```python
from build123d import *

# Parameters (mm, degrees)
SKETCH1_W           = 120
SKETCH1_H           = 20
SKETCH1_W_2         = 25.5
SKETCH1_H_2         = 12.4
BOSS_EXTRUDE1_DEPTH = 6
SKETCH3_R           = 0.55
BOSS_EXTRUDE2_DEPTH = 3
SKETCH4_W           = 36
SKETCH4_H           = 20
BOSS_EXTRUDE3_DEPTH = 1.8
SKETCH5_R           = 3.4
CUT_EXTRUDE1_DEPTH  = 1.8
FILLET1_R           = 0.6


with BuildPart() as part:
    # Sketch1 → Boss-Extrude1 (new body)
    with BuildSketch(Plane(origin=(0, 0, 0), x_dir=(1, 0, 0), z_dir=(0, 1, 0))):
        with Locations((60, 10)):
            Rectangle(SKETCH1_W, SKETCH1_H)
        with BuildLine():
            Line((93.674922601, 11.942124585), (109.694736842, 13.386268507))
            ThreePointArc((109.694736842, 13.386268507), (113.4, 10), (109.694736842, 6.613731493))
            Line((109.694736842, 6.613731493), (93.674922601, 8.057875415))
            ThreePointArc((93.674922601, 8.057875415), (91.9, 10), (93.674922601, 11.942124585))
        make_face(mode=Mode.SUBTRACT)
        with Locations((17.75, 10)):
            Rectangle(SKETCH1_W_2, SKETCH1_H_2, mode=Mode.SUBTRACT)
    extrude(amount=BOSS_EXTRUDE1_DEPTH)

    # Sketch3 → Boss-Extrude2 (add)
    with BuildSketch(Plane.XZ):
        with Locations(Location((4.25, -10, 0), (0, 0, 270))):
            Circle(SKETCH3_R)
        with Locations(Location((31.25, -10, 0), (0, 0, 270))):
            Circle(SKETCH3_R)
    extrude(amount=BOSS_EXTRUDE2_DEPTH)

    # Sketch4 → Boss-Extrude3 (add)
    with BuildSketch(Plane(origin=(0, 6, 0), x_dir=(1, 0, 0), z_dir=(0, 1, 0))):
        with Locations((102, 10)):
            Rectangle(SKETCH4_W, SKETCH4_H)
    extrude(amount=-BOSS_EXTRUDE3_DEPTH)

    # Sketch5 → Cut-Extrude1 (cut)
    with BuildSketch(Plane.XZ.offset(-4.2)):
        with Locations(Location((110, -10, 0), (0, 0, 270))):
            Circle(SKETCH5_R)
    extrude(amount=-CUT_EXTRUDE1_DEPTH, mode=Mode.SUBTRACT)

    # Fillet1
    fillet1_edges = [part.edges().sort_by_distance(p)[0] for p in [
        (120, 6, -10),
        (60, 6, -20),
        (0, 6, -10),
        (60, 0, -20),
        (120, 0, -10),
        (60, 0, 0),
        (0, 0, -10),
        (60, 6, 0),
    ]]
    fillet(fillet1_edges, radius=FILLET1_R)


solid = part.part
```
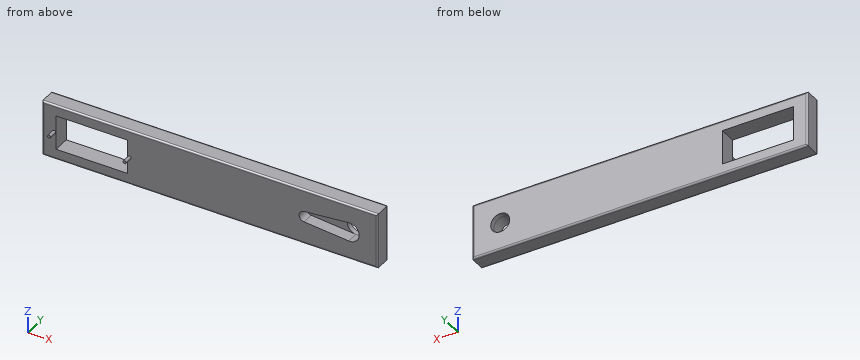
For this review, take the finished solid that the model builds, in its own axes (mm). Coordinates: 2 decimals unless noted, no trailing zeros. Order: outer loops, then holes, each group sorted by start corner. A loop starts at its lowest first (then second) coordinate and runs counter-clockwise, first axis right, second up. Notation, with made-up numbers: (-19, 66.25) -> (-4, 66.25) arc R12 ccw to (-4, 85.25) -> close; hole circle Ø10 at (-5, -13). An arc over 180 degrees is marked (long way). Answer as CSV lines item,"result".
Q1. Clearance check with a flat-ended pin moving along its axis: pin 1 Ø3.5 at (x, z) = (103.5, -11) entering from -Y. State where the tip first meets the part, or that it passes through.
Model answer:
pin 1,"stops at y = 4.2"
Q2. We need section B-B (x = 57). State the section outline as (y, z) points.
Model answer:
outline,"(0, -19.4) arc R0.6 ccw to (0.6, -20) -> (5.4, -20) arc R0.6 ccw to (6, -19.4) -> (6, -0.6) arc R0.6 ccw to (5.4, 0) -> (0.6, 0) arc R0.6 ccw to (0, -0.6) -> close"
Q3. We need section A-A (y = 2). State the section outline as (x, z) points.
Model answer:
outline,"(0, -20) -> (120, -20) -> (120, 0) -> (0, 0) -> close; hole (5, -16.2) -> (30.5, -16.2) -> (30.5, -3.8) -> (5, -3.8) -> close; hole (93.67, -11.94) -> (109.69, -13.39) arc R3.4 ccw (long way) to (109.69, -6.61) -> (93.67, -8.06) arc R1.95 ccw to start"
Q4. Wall thickness on line 1 along X through (y, z) = (2.6, -10); line 2 along X through (y, z) = (4.9, -10); line 3 along X through (y, z) = (3.25, -4.75): over which ranges is each line inside the solid? List them lowest first. Write a range as [from, to].
Model answer:
line 1,"x = [0, 5], [30.5, 91.9], [113.4, 120]"
line 2,"x = [0, 5], [30.5, 106.6], [113.4, 120]"
line 3,"x = [0, 5], [30.5, 120]"
